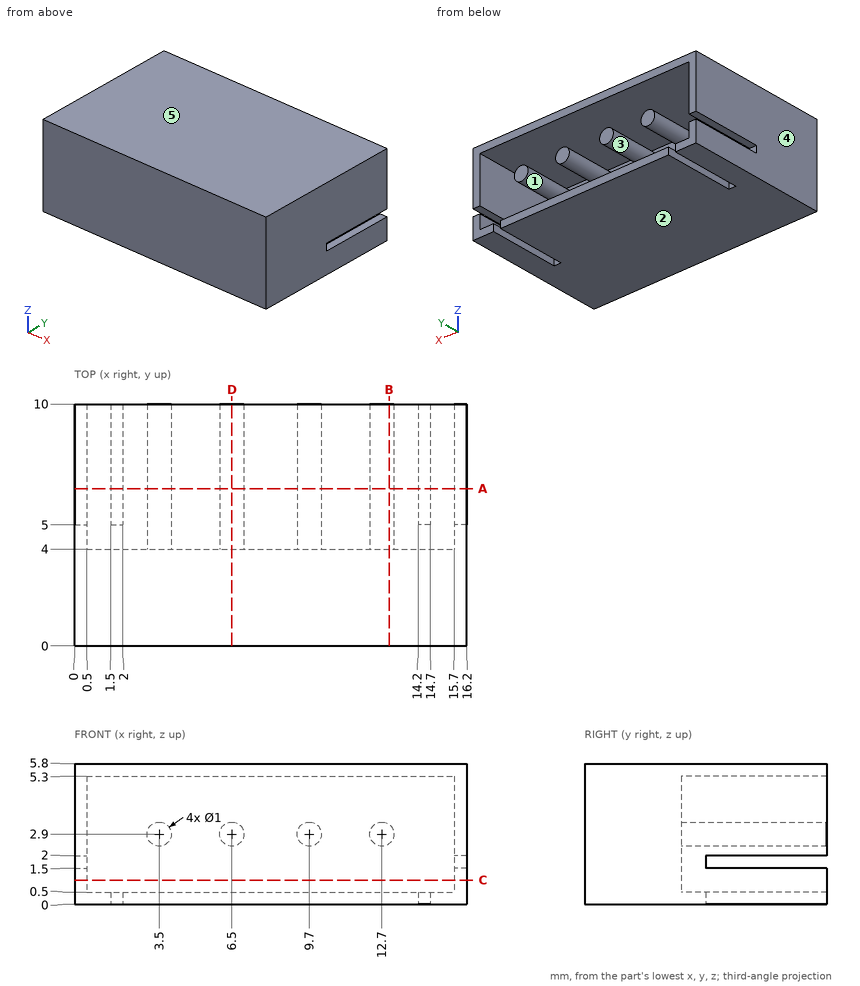
Answer from the drawing. Dimensions are ordinates in mm from the lowest x, y and z of the part. A direction names the side the tool comes from. Round coordinates to 2 decimals unless told otherwise and drop trailing zeros. Loops run counter-clockwise (first coordinate to the right, second up) from the corner with the lowest first, then second, coordinate; pieces in that order, holes last. Notation, with made-up numbers: (19, -39) - (50, -39) arc R22 ccw to (50, 0) - close; hole circle Ø6 at (80.25, 3.25). An arc over 180 degrees is marked (long way). Return JSON: item names as keys, results as strings. Group by question number.
1. The part is cut by section A-A on y = 6.5. Determine the outline of the cut face in (x, z).
2. The part is cut by section B-B on x = 13. Determine the outline of the cut face in (y, z).
3. Which of the six approach directions +Z, -Z, +X, -X, +Y, -Y give full straight-line access (tool end or side, diameter ignored) to the marked faces 1 and 2?
4. Consider probe 1 along X at (y, z) = (7, 2.2); probe 2 along Z at (x, y) = (1, 8.75); probe 3 along X at (y, z) = (5.25, 2.65). Determine where each line is inside the solid, lowest interval first.
5. The part is cut by section D-D on x = 6.5. Determine the outline of the cut face in (y, z).
6. The part is cut by section C-C on z = 1. Determine the outline of the cut face in (x, y), then the cut area to 3 significant figures.
7. The mould has two halves that part along Z. Classify the marked faces 3, 4 and 5: pulls with the +Z half, pulls with the -Z half, needs draft (parallel to the pull), parting line crosses it, or undercut.
8. This flat-tipped pin is pushed along its axis until it touches: P1, Ø0.6, axis at x = 0.5, y = 8.5, coming from the -Z side. Where does it stop, or does it pass through?
Resolved:
{
 "1": {"outline": "(0, 0) - (1.5, 0) - (1.5, 0.5) - (0.5, 0.5) - (0.5, 1.5) - (0, 1.5) - close; (0, 2) - (0.5, 2) - (0.5, 5.3) - (15.7, 5.3) - (15.7, 2) - (16.2, 2) - (16.2, 5.8) - (0, 5.8) - close; (2, 0) - (14.2, 0) - (14.2, 0.5) - (2, 0.5) - close; circle Ø1 at (3.5, 2.9); circle Ø1 at (6.5, 2.9); circle Ø1 at (9.7, 2.9); circle Ø1 at (12.7, 2.9); (14.7, 0) - (16.2, 0) - (16.2, 1.5) - (15.7, 1.5) - (15.7, 0.5) - (14.7, 0.5) - close"},
 "2": {"outline": "(0, 0) - (10, 0) - (10, 0.5) - (4, 0.5) - (4, 2.5) - (10, 2.5) - (10, 3.3) - (4, 3.3) - (4, 5.3) - (10, 5.3) - (10, 5.8) - (0, 5.8) - close"},
 "3": {"face 1": "+Y", "face 2": "-Z, +X, -X, +Y, -Y"},
 "4": {"probe 1": "x = 0 to 0.5, 15.7 to 16.2", "probe 2": "z = 0 to 0.5, 5.3 to 5.8", "probe 3": "x = 0 to 0.5, 3.07 to 3.93, 6.07 to 6.93, 9.27 to 10.13, 12.27 to 13.13, 15.7 to 16.2"},
 "5": {"outline": "(0, 0) - (10, 0) - (10, 0.5) - (4, 0.5) - (4, 2.4) - (10, 2.4) - (10, 3.4) - (4, 3.4) - (4, 5.3) - (10, 5.3) - (10, 5.8) - (0, 5.8) - close"},
 "6": {"outline": "(0, 0) - (16.2, 0) - (16.2, 10) - (15.7, 10) - (15.7, 4) - (0.5, 4) - (0.5, 10) - (0, 10) - close", "area": "70.8 mm²"},
 "7": {"face 3": "undercut", "face 4": "needs draft", "face 5": "pulls with the +Z half"},
 "8": {"P1": "stops at z = 0"}
}
